```python
from build123d import *

# Parameters (mm, degrees)
SKETCH_1_W          = 130
SKETCH_1_H          = 40
EXTRUDE_1_DEPTH     = 10
SKETCH_2_W          = 100
SKETCH_2_H          = 40
EXTRUDE_2_DEPTH     = 20
SKETCH_3_R          = 6
CUT_EXTRUDE_1_DEPTH = 20
SKETCH_4_R          = 4
CUT_EXTRUDE_2_DEPTH = 75.330343737


with BuildPart() as part:
    # 草图1 → 凸台-拉伸1 (new body)
    with BuildSketch(Plane(origin=(0, 0, 0), x_dir=(1, 0, 0), z_dir=(0, 1, 0))):
        Rectangle(SKETCH_1_W, SKETCH_1_H)
    extrude(amount=EXTRUDE_1_DEPTH)

    # 草图2 → 凸台-拉伸2 (add)
    with BuildSketch(Plane(origin=(0, 10, 0), x_dir=(1, 0, 0), z_dir=(0, 1, 0))):
        Rectangle(SKETCH_2_W, SKETCH_2_H)
    extrude(amount=EXTRUDE_2_DEPTH)

    # 草图3 → 切除-拉伸1 (cut)
    with BuildSketch(Plane(origin=(0, 30, 0), x_dir=(1, 0, 0), z_dir=(0, 1, 0))):
        with Locations(Location((-33, 0, 0), (0, 0, 270))):
            Circle(SKETCH_3_R)
        with Locations(Location((-11, 0, 0), (0, 0, 270))):
            Circle(SKETCH_3_R)
        with Locations(Location((11, 0, 0), (0, 0, 270))):
            Circle(SKETCH_3_R)
        with Locations(Location((33, 0, 0), (0, 0, 270))):
            Circle(SKETCH_3_R)
    extrude(amount=-CUT_EXTRUDE_1_DEPTH, mode=Mode.SUBTRACT)

    # 草图4 → 切除-拉伸2 (cut, through all)
    with BuildSketch(Plane(origin=(0, 30, 0), x_dir=(1, 0, 0), z_dir=(0, 1, 0))):
        with Locations(Location((-57.5, 0, 0), (0, 0, 270))):
            Circle(SKETCH_4_R)
        with Locations(Location((57.5, 0, 0), (0, 0, 270))):
            Circle(SKETCH_4_R)
    extrude(amount=-CUT_EXTRUDE_2_DEPTH, mode=Mode.SUBTRACT)


solid = part.part
```
Source: CAD feature listing. Evaluate the final solid. Frame: model axes, mm. A direction names the side the tool comes from. Give positions to 0.01 mm unless a question says otherwise; leave off trailing zeros. Write each loop counter-clockwise with the first axis right and the second up, starting at its lowest first coordinate (ties: lowest second). Pieces come first, ordered by that corner, then holes.
1. Access query for faces 1 (the face through (-50, 20, 0)), 2 (the face through (-5.05, 20.14, -0.78)), 3 (the face through (-1, 0, 0)), 4 (the face through (57.4, 10, 4.2)). Directions: +Z, -Z, +X, -X, +Y, -Y. A direction counts if a zero-diameter tool reaches every point of the face in a straight line with its end or side. Return the directions, or none.
2. Material intervals for line 1 along X through (y, z) = (20.25, 0); line 2 along X through (y, z) = (3, 0); line 3 along X through (y, z) = (24, 2.5), sorted ascending.
3. Section query D-D (z = 11). Return the cut outline in (x, y), then the cut area to 3 significant figures.
4. Pull-direction query (X, two-part tool) for faces 5 (the face through (-1, 30, 0)), 6 (the face through (-33, 10, 0)), 7 (the face through (50, 20, 0)), 8 (the face through (-65, 5, 0)); classes: +X half, -X half, draft (parallel to the pull), parting line (faces both ways), or undercut.
5. First-contact query: pin 1 (12 mm diameter, centred on y = 18, z = 14, fed in from -X); pin 2 (12 mm diameter, centred on x = -58, z = -1.5, fed in from +Y). Flat tips, straight axial feed; report the tip coordinate or a pass-through.
6. Section query C-C (y = 21.5). Return the cut outline in (x, z), then the cut area to 3 significant figures.
7. Section query A-A (x = -57.5). Return the cut outline in (y, z), then the cut area to 3 significant figures.
8. Section query B-B (z = -2). Count the separate pieces of the cut face and the enclosed holes in it, then the cut area to 3 significant figures.
Output values:
1. face 1: +Z, -Z, -X, +Y
1. face 2: +Y
1. face 3: +Z, -Z, +X, -X, -Y
1. face 4: +Z, -Z, +X, +Y
2. line 1: x = -50 to -39, -27 to -17, -5 to 5, 17 to 27, 39 to 50
2. line 2: x = -65 to -61.5, -53.5 to 53.5, 61.5 to 65
2. line 3: x = -50 to -38.45, -27.55 to -16.45, -5.55 to 5.55, 16.45 to 27.55, 38.45 to 50
3. outline: (-65, 0) - (65, 0) - (65, 10) - (50, 10) - (50, 30) - (-50, 30) - (-50, 10) - (-65, 10) - close
3. area: 3,300 mm2
4. face 5: draft
4. face 6: undercut
4. face 7: +X half
4. face 8: -X half
5. pin 1: stops at x = -50
5. pin 2: stops at y = 10
6. outline: (-50, -20) - (50, -20) - (50, 20) - (-50, 20) - close; hole circle Ø12 at (-33, 0); hole circle Ø12 at (-11, 0); hole circle Ø12 at (11, 0); hole circle Ø12 at (33, 0)
6. area: 3,550 mm2
7. outline: (0, -20) - (10, -20) - (10, -4) - (0, -4) - close; (0, 4) - (10, 4) - (10, 20) - (0, 20) - close
7. area: 320 mm2
8. separate pieces: 3
8. enclosed holes: 0
8. area: 2,260 mm2
